Part model, mm, in its own coordinate system. Face numbers are marked on the shaded views. A direction names the side the tool comes from. Round coordinates to 2 decimals unless told otherwise and drop trailing zeros. Write each loop counter-clockwise with the first axis right and the second up, starting at its lowest first coordinate (ties: lowest second). Pieces come first, ordered by that corner, then holes.
Autodesk Fusion 360 part; units mm, degrees
sketch "Sketch1" plane through (0, 0, 0) normal (0, 0, 1) x (1, 0, 0)
  line L0 (0, 0) -> (50, 0)
  line L1 (50, 0) -> (50, 80)
  line L2 (50, 80) -> (0, 80)
  line L3 (0, 80) -> (0, 0)
  dimension "d1" = 50
  dimension "d2" = 80
extrude "Extrude1" add sketch "Sketch1" along normal blind 5
sketch "Sketch2" plane through (0, 0, 5) normal (0, 0, 1) x (-1, 0, 0)
  line L0 (0, -80) -> (0, 0)
  line L1 (0, 0) -> (-50, 0)
  line L2 (-50, 0) -> (-50, -80)
  line L3 (-50, -80) -> (0, -80)
  line L4 (-40, -10) -> (-10, -10)
  line L5 (-10, -10) -> (-10, -70)
  line L6 (-10, -70) -> (-40, -70)
  line L7 (-40, -70) -> (-40, -10)
  line L8 (-40, -10) -> (-10, -70) construction
  line L9 (-10, -10) -> (-40, -70) construction
  point P0 (-25, -40)
  point P1 (-25, -40)
  dimension "d5" = 30
  dimension "d6" = 60
extrude "Extrude2" cut sketch "Sketch2" against normal blind 6 contours L4 L5 L6 L7
sketch "Sketch3" plane through (0, 0, 5) normal (0, 0, 1) x (-1, 0, 0)
  line L0 (-10, -10) -> (-10, -70)
  line L1 (-10, -70) -> (-40, -70)
  line L2 (-40, -70) -> (-40, -10)
  line L3 (-40, -10) -> (-10, -10)
  line L4 (0, -80) -> (0, 0)
  line L5 (0, 0) -> (-50, 0)
  line L6 (-50, 0) -> (-50, -80)
  line L7 (-50, -80) -> (0, -80)
  point P0 (-25, -76)
  point P1 (-25, -4)
hole "Hole1" at (25, 76, 5) at (25, 4, 5) direction (0, 0, -1) diameter 2.75 depth 15 tip angle 118
sketch "Sketch4" plane through (0, 0, 0) normal (0, 0, -1) x (1, 0, 0)
  circle A0 centre (25, -76) radius 1.375
  circle A1 centre (25, -4) radius 1.375
  line L0 (10, -70) -> (10, -10)
  line L1 (10, -10) -> (40, -10)
  line L2 (40, -10) -> (40, -70)
  line L3 (40, -70) -> (10, -70)
  line L4 (0, 0) -> (0, -80)
  line L5 (0, -80) -> (50, -80)
  line L6 (50, -80) -> (50, 0)
  line L7 (50, 0) -> (0, 0)
  line L8 (48, -2) -> (2, -2)
  line L9 (2, -2) -> (2, -78)
  line L10 (2, -78) -> (48, -78)
  line L11 (48, -78) -> (48, -2)
extrude "Extrude3" add sketch "Sketch4" along normal blind 80 contours L4 L5 L6 L7
sketch "Sketch5" plane through (0, 0, 0) normal (-1, 0, 0) x (0, -1, 0)
  line L0 (0, -80) -> (0, 5)
  line L1 (0, 5) -> (-80, 5)
  line L2 (-80, 5) -> (-80, -80)
  line L3 (-80, -80) -> (0, -80)
  point P0 (-10, -5)
  point P1 (-70, -5)
hole "Hole2" at (0, 10, -5) at (0, 70, -5) direction (1, 0, 0) diameter 5.5 depth 100 tip angle 118
sketch "Sketch6" plane through (0, 80, 0) normal (0, 1, 0) x (-1, 0, 0)
  line L0 (0, -80) -> (0, 5)
  line L1 (0, 5) -> (-50, 5)
  line L2 (-50, 5) -> (-50, -80)
  line L3 (-50, -80) -> (0, -80)
  point P0 (-10, -5)
  point P1 (-40, -5)
hole "Hole3" at (40, 80, -5) at (10, 80, -5) direction (0, -1, 0) diameter 5.5 depth 100 tip angle 118
sketch "Sketch7" plane through (0, 78, 0) normal (0, -1, 0) x (1, 0, 0)
  circle A0 centre (40, -5) radius 2.75
  circle A1 centre (10, -5) radius 2.75
  line L0 (48, 0) -> (2, 0)
  line L1 (2, 0) -> (2, -80)
  line L2 (2, -80) -> (48, -80)
  line L3 (48, -80) -> (48, 0)
  line L4 (30, -80) -> (20, -80)
  line L5 (20, -80) -> (20, -70)
  line L6 (20, -70) -> (30, -70)
  line L7 (30, -70) -> (30, -80)
  dimension "d20" = 10
  dimension "d21" = 10
extrude "Extrude4" add sketch "Sketch7" along normal blind 10 contours L2 L4 L5 L6 L7
sketch "Sketch8" plane through (0, 2, 0) normal (0, 1, 0) x (-1, 0, 0)
  circle A0 centre (-40, -5) radius 2.75
  circle A1 centre (-10, -5) radius 2.75
  line L0 (-2, 0) -> (-48, 0)
  line L1 (-48, 0) -> (-48, -80)
  line L2 (-48, -80) -> (-2, -80)
  line L3 (-2, -80) -> (-2, 0)
  line L4 (-20, -80) -> (-30, -80)
  line L5 (-30, -80) -> (-30, -70)
  line L6 (-30, -70) -> (-20, -70)
  line L7 (-20, -70) -> (-20, -80)
  dimension "d24" = 10
  dimension "d25" = 10
extrude "Extrude5" add sketch "Sketch8" along normal blind 10 contours L2 L4 L5 L6 L7
sketch "Sketch9" plane through (0, 0, -80) normal (0, 0, -1) x (1, 0, 0)
  line L0 (48, -2) -> (48, -78)
  line L1 (48, -78) -> (30, -78)
  line L2 (30, -78) -> (30, -68)
  line L3 (30, -68) -> (20, -68)
  line L4 (20, -68) -> (20, -78)
  line L5 (20, -78) -> (2, -78)
  line L6 (2, -78) -> (2, -2)
  line L7 (2, -2) -> (20, -2)
  line L8 (20, -2) -> (20, -12)
  line L9 (20, -12) -> (30, -12)
  line L10 (30, -12) -> (30, -2)
  line L11 (30, -2) -> (48, -2)
  line L12 (50, 0) -> (0, 0)
  line L13 (0, 0) -> (0, -80)
  line L14 (0, -80) -> (50, -80)
  line L15 (50, -80) -> (50, 0)
  line L16 (1, -1) -> (49, -1)
  line L17 (49, -1) -> (49, -79)
  line L18 (49, -79) -> (1, -79)
  line L19 (1, -79) -> (1, -1)
extrude "Extrude6" cut sketch "Sketch9" against normal blind 2 contours L16 L17 L18 L19
sketch "Sketch10" plane through (0, 0, -78) normal (0, 0, -1) x (1, 0, 0)
  line L0 (30, -12) -> (30, -2)
  line L1 (30, -2) -> (48, -2)
  line L2 (48, -2) -> (48, -78)
  line L3 (48, -78) -> (30, -78)
  line L4 (30, -78) -> (30, -68)
  line L5 (30, -68) -> (20, -68)
  line L6 (20, -68) -> (20, -78)
  line L7 (20, -78) -> (2, -78)
  line L8 (2, -78) -> (2, -2)
  line L9 (2, -2) -> (20, -2)
  line L10 (20, -2) -> (20, -12)
  line L11 (20, -12) -> (30, -12)
  line L12 (1, -79) -> (49, -79)
  line L13 (49, -79) -> (49, -1)
  line L14 (49, -1) -> (1, -1)
  line L15 (1, -1) -> (1, -79)
  point P0 (25, -7)
  point P1 (25, -73)
hole "Hole4" at (25, 7, -78) at (25, 73, -78) direction (0, 0, 1) diameter 2.75 depth 11 tip angle 180
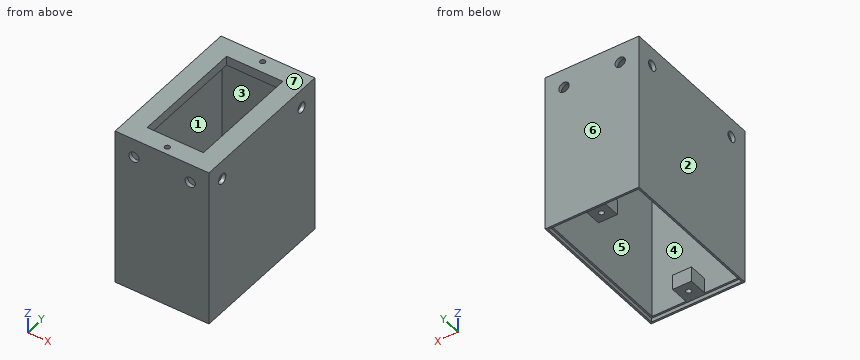
Q1. Wall check: L1, parallel to X at y = 73, z = -75 (3 decimals); L2, parallel to X at y = 79, z = -5; L3, parallel to Y at x = 48.7, z = -5. Give the ranges that are in metal, low to high.
Values follow:
L1: x = 0 to 2, 20 to 23.625, 26.375 to 30, 48 to 50
L2: x = 0 to 7.25, 12.75 to 37.25, 42.75 to 50
L3: y = 0 to 7.25, 12.75 to 67.25, 72.75 to 80
Q2. Drop a flat-ended pin along its axis: pin 1 (2 mm diameter, centred on x = 25, y = 76, fed in from +Z). Give the stop position or say it passes through.
Values follow:
pin 1: stops at z = -70
Q3. Cut at B-B on z = -44. Write the cut outline in (x, y), plus the area to 3 significant figures.
Values follow:
outline: (0, 0) - (50, 0) - (50, 80) - (0, 80) - close; hole (2, 2) - (48, 2) - (48, 78) - (2, 78) - close
area: 504 mm2
Q4. Which spindle directions (+Z, -Z, +X, -X, +Y, -Y) get a long thin tool onto all of the face, cutting with end or side? Do the marked faces 1, 2 and 3. Say none if no direction does.
Values follow:
face 1: -Z
face 2: +Z, -Z, -X, +Y, -Y
face 3: none
Q5. Mould opens along Y. For the marked faces 4, 5, 6 and 7 say: +Y half, -Y half, draft (parallel to the pull), parting line (faces both ways), or undercut.
Values follow:
face 4: undercut
face 5: undercut
face 6: +Y half
face 7: draft
Q6. Cut at D-D on z = -73. Write the cut outline in (x, y) (3 decimals).
Values follow:
outline: (0, 0) - (50, 0) - (50, 80) - (0, 80) - close; hole (2, 2) - (20, 2) - (20, 12) - (30, 12) - (30, 2) - (48, 2) - (48, 78) - (30, 78) - (30, 68) - (20, 68) - (20, 78) - (2, 78) - close; hole circle Ø2.75 at (25, 7); hole circle Ø2.75 at (25, 73)
Q7. Cut at A-A on x = 36. Write the cut outline in (y, z), plus the area to 3 significant figures.
Values follow:
outline: (0, -80) - (1, -80) - (1, -78) - (2, -78) - (2, 0) - (10, 0) - (10, 5) - (0, 5) - close; (70, 0) - (78, 0) - (78, -78) - (79, -78) - (79, -80) - (80, -80) - (80, 5) - (70, 5) - close
area: 416 mm2
Q8. Cut at C-C on y = 38. Write the cut outline in (x, z), plus the area to 3 significant figures.
Values follow:
outline: (0, -80) - (1, -80) - (1, -78) - (2, -78) - (2, 0) - (10, 0) - (10, 5) - (0, 5) - close; (40, 0) - (48, 0) - (48, -78) - (49, -78) - (49, -80) - (50, -80) - (50, 5) - (40, 5) - close
area: 416 mm2
